Part model, mm, in its own coordinate system. Face numbers are marked on the shaded views. A direction names the side the tool comes from. Round coordinates to 2 decimals unless told otherwise and drop trailing zeros. Loops run counter-clockwise (first coordinate to the right, second up) from the corner with the lowest first, then second, coordinate; pieces in that order, holes last.
(1) Cut at B-B on y = -5.25. List the corners of the cut face in (x, z).
(2) Cut at C-C on z = -3.5. List the corners of the cut face in (x, y).
(3) Tool access for the marked faces 1, 2 and 3: list every direction of +Z, -Z, +X, -X, +Y, -Y with a clear straight run to the whole face (end or side of a thin tool).
(4) Flat gauge pins, fed straight in: pin 1 (10 mm diameter, centred on x = -28, z = 8.5, fed in from +Y); pin 2 (6.5 mm diameter, centred on x = 26, y = 3.5, fed in from +Z); pin 3 (10 mm diameter, centred on x = -30, z = 8, fed in from -Y). Where does each tip first touch, or does it go through?
(5) Cut at A-A on x = -24. List the corners of the cut face in (y, z).
(6) Mould opens along Y. For the marked faces 4, 5 and 6 say: +Y half, -Y half, draft (parallel to the pull), parting line (faces both ways), or undercut.
(7) Cut at D-D on z = 4. List the corners of the cut face in (x, y), then the cut area to 3 significant figures.
(8) Probe probe 1 along Y at (x, z) = (36, -5.5); probe 2 along Z at (x, y) = (31, -8.75); probe 3 along X at (y, z) = (-9.5, -2). List the from-to ranges inside material, lowest first.
from build123d import *

# Parameters (mm, degrees)
SKETCH1_W                = 100
SKETCH1_H                = 25
BOSS_EXTRUDE1_DEPTH      = 14.1675
BOSS_EXTRUDE2_DEPTH      = 12.7325
BOSS_EXTRUDE2_DEPTH_BACK = 11.1675
FILLET1_R                = 2
CUT_EXTRUDE1_DEPTH       = 12.7325
CUT_EXTRUDE1_DEPTH_BACK  = 11.1675
FILLET2_R                = 2


with BuildPart() as part:
    # Sketch1 → Boss-Extrude1 (new, symmetric)
    with BuildSketch(Plane(origin=(0, 0, 0), x_dir=(1, 0, 0), z_dir=(0, 1, 0))):
        with Locations((0, 12.5)):
            Rectangle(SKETCH1_W, SKETCH1_H)
    extrude(amount=BOSS_EXTRUDE1_DEPTH, both=True)

    # Sketch2 → Boss-Extrude2 (add, two sides: drawn at the far end of the back side and taken through both)
    with BuildSketch(Plane(origin=(0, 0, 0), x_dir=(1, 0, 0), z_dir=(0, 1, 0)).offset(-BOSS_EXTRUDE2_DEPTH_BACK)):
        Polygon((-43.283333333, 0), (-13.283333333, 0), (-20.500211698, -12.5), (-36.066454968, -12.5), align=None)
    extrude(amount=BOSS_EXTRUDE2_DEPTH + BOSS_EXTRUDE2_DEPTH_BACK)

    # Fillet1
    fillet1_edges = [part.edges().sort_by_distance(p)[0] for p in [
        (-20.500211698, 0.7825, 12.5),
        (-36.066454968, 0.7825, 12.5),
    ]]
    fillet(fillet1_edges, radius=FILLET1_R)

    # Sketch2<3> → Cut-Extrude1 (cut, two sides: drawn at the far end of the back side and taken through both)
    with BuildSketch(Plane(origin=(0, 0, 0), x_dir=(1, 0, 0), z_dir=(0, 1, 0)).offset(-CUT_EXTRUDE1_DEPTH_BACK)):
        Polygon((36.066454968, 12.5), (20.500211698, 12.5), (13.283333333, 0), (43.283333333, 0), align=None)
    extrude(amount=CUT_EXTRUDE1_DEPTH + CUT_EXTRUDE1_DEPTH_BACK, mode=Mode.SUBTRACT)

    # Fillet2
    fillet2_edges = [part.edges().sort_by_distance(p)[0] for p in [
        (36.066454968, 0.7825, -12.5),
        (20.500211698, 0.7825, -12.5),
    ]]
    fillet(fillet2_edges, radius=FILLET2_R)


solid = part.part
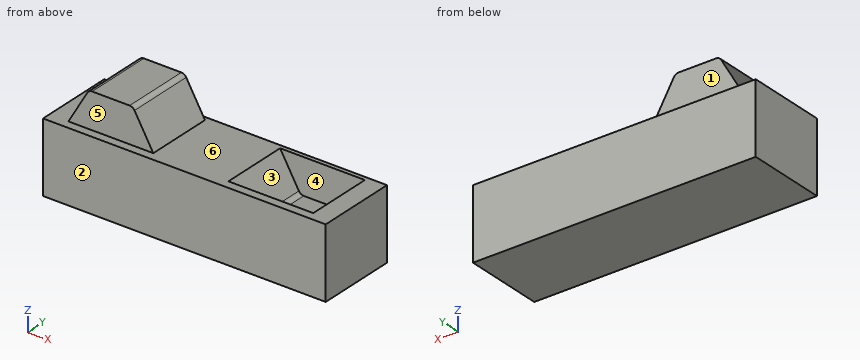
Final values:
1. outline: (-50, -25) - (50, -25) - (50, 0) - (43.28, 0) - (36.64, -11.5) arc R2 cw to (34.91, -12.5) - (21.65, -12.5) arc R2 cw to (19.92, -11.5) - (13.28, 0) - (-13.28, 0) - (-19.92, 11.5) arc R2 ccw to (-21.65, 12.5) - (-34.91, 12.5) arc R2 ccw to (-36.64, 11.5) - (-43.28, 0) - (-50, 0) - close
2. outline: (-50, -14.17) - (50, -14.17) - (50, 14.17) - (-50, 14.17) - close; hole (15.3, -11.17) - (41.26, -11.17) - (41.26, 12.73) - (15.3, 12.73) - close
3. face 1: +Z, +X, -X, +Y
3. face 2: +Z, -Z, +X, -X, -Y
3. face 3: +Z
4. pin 1: stops at y = 12.73
4. pin 2: stops at z = -12.5
4. pin 3: stops at y = -11.17
5. outline: (-14.17, -25) - (14.17, -25) - (14.17, 0) - (12.73, 0) - (12.73, 12.5) - (-11.17, 12.5) - (-11.17, 0) - (-14.17, 0) - close
6. face 4: undercut
6. face 5: -Y half
6. face 6: draft
7. outline: (-40.97, -11.17) - (-15.59, -11.17) - (-15.59, 12.73) - (-40.97, 12.73) - close
7. area: 607 mm2
8. probe 1: y = -14.17 to -11.17, 12.73 to 14.17
8. probe 2: z = -25 to -12.5
8. probe 3: x = -50 to 14.44, 42.13 to 50
